The listing builds one solid part. Answer for the finished solid, in the listing's coordinates (mm). A direction names the side the tool comes from. Give positions to 0.01 mm unless a question says otherwise; leave off trailing zeros. Order: outer loops, then holes, each group sorted by start corner. A loop starts at its lowest first (then second) coordinate and runs counter-clockwise, first axis right, second up. Notation, with made-up numbers: (58.25, -19.75) - (112.25, -19.75) arc R25 cw to (112.25, -4.75) - close; hole circle Ø1 at (-14.5, 49.5). An arc over 180 degrees is marked (long way). Write each question's results on one line, items separated by ' | '. Start each with the question number.
1. Determine the mould class of faces 6 (the face through (-69.52, 2.54, 69.82)), 7 (the face through (-67.114, -30, 90)), 8 (the face through (-89, -30, 64.614)) for opening direction Z: released by +Z, released by -Z, zero draft, split by the parting line, or undercut.
2. Which of the six approach directions +Z, -Z, +X, -X, +Y, -Y give full straight-line access (tool end or side, diameter ignored) to faces 1 (the face through (-90, -10, 64.614)), 2 (the face through (-69.36, -9.96, 69.49)), 3 (the face through (-60.858, -18, 91)), 4 (the face through (-46.49, 10.21, 60.63)), 5 (the face through (-64.614, -10, 90))?
3. Section C-C (x = -91) is taken. Give the vertices of the cut face in (y, z).
4. Find the intervals of material crossed by L1, parallel to X at y = -10, z = 94; L2, parallel to Y at x = -71, z = 94; L3, parallel to Z at x = -98, y = -3, in increasing order.
5. Flat-ended cylindrical pins translate along their axes: pin 1 (6 mm diameter, centred on y = 4.5, z = 92, fed in from +X); pin 2 (10 mm diameter, centred on y = 3.5, z = 67.5, fed in from +X); pin 3 (5 mm diameter, centred on y = -10, z = 97.5, fed in from -X); pin 4 (3 mm diameter, centred on x = -89.5, y = -29.5, fed in from -Z). Find the tip coordinate at first contact, or state that the pin passes through.
6. Section D-D (z = 81) is taken. Give the vertices of the cut face in (x, y).
7. Section B-B (z = 96.5) is taken. Give the vertices of the cut face in (x, y), and give its area (3 significant figures).
8. Section A-A (y = -29) is taken. Give the vertices of the cut face in (x, z), and give its area (3 significant figures).
from build123d import *

# Parameters (mm, degrees)
BOSS_EXTRUDE1_DEPTH     = 30
SKETCH2_R               = 2.8
CUT_EXTRUDE1_DEPTH      = 65
CUT_EXTRUDE2_DEPTH      = 65
BOSS_EXTRUDE2_DEPTH     = 40
SKETCH9_W               = 55.910316486
SKETCH9_H               = 20
CUT_EXTRUDE4_DEPTH      = 40
CUT_EXTRUDE5_DEPTH      = 40
CHAMFER1_SIZE           = 5
CUT_EXTRUDE6_DEPTH      = 3
CUT_EXTRUDE6_DEPTH_BACK = 3
CUT_EXTRUDE7_DEPTH      = 3
CUT_EXTRUDE7_DEPTH_BACK = 3
SKETCH14_W              = 8
SKETCH14_H              = 30
BOSS_EXTRUDE3_DEPTH     = 2
CUT_EXTRUDE8_DEPTH      = 22
CHAMFER2_SIZE           = 2


with BuildPart() as part:
    # Sketch1 → Boss-Extrude1 (new body)
    with BuildSketch(Plane(origin=(0, 0, 0), x_dir=(1, 0, 0), z_dir=(0, 1, 0))):
        Polygon((-69, -54.857864376), (-54.857864376, -69), (-39.30151519, -53.443650814), (-33.644660941, -59.100505063), (-49.544155877, -75), (-75, -75), (-75, -49.544155877), (-59.100505063, -33.644660941), (-53.443650814, -39.30151519), align=None)
    extrude(amount=BOSS_EXTRUDE1_DEPTH)

    # Sketch2 → Cut-Extrude1 (cut)
    with BuildSketch(Plane(origin=(12.727922061, 0, 12.727922061), x_dir=(0.707106781, 0, -0.707106781), z_dir=(0.707106781, 0, 0.707106781))):
        with Locations((-70.580735804, 15)):
            Circle(SKETCH2_R)
    extrude(amount=-CUT_EXTRUDE1_DEPTH, mode=Mode.SUBTRACT)

    # Sketch4 → Cut-Extrude2 (cut)
    with BuildSketch(Plane.XZ):
        Polygon((-60.857864376, 75), (-75, 60.857864376), (-82.434342637, 68.292207014), (-68.292207014, 82.434342637), align=None)
    extrude(amount=-CUT_EXTRUDE2_DEPTH, mode=Mode.SUBTRACT)

    # Sketch6 → Boss-Extrude2 (add)
    with BuildSketch(Plane.XZ):
        Polygon((-60.857864376, 75), (-60.857864376, 105.632615689), (-75, 105.632615689), (-75, 75), (-104.149605391, 75), (-104.149605391, 60.857864376), (-75, 60.857864376), (-75, 49.544155877), (-59.100505063, 33.644660941), (-53.443650814, 39.30151519), (-69, 54.857864376), (-54.857864376, 69), (-39.30151519, 53.443650814), (-33.644660941, 59.100505063), (-49.544155877, 75), align=None)
    extrude(amount=BOSS_EXTRUDE2_DEPTH)

    # Sketch9 → Cut-Extrude4 (cut)
    with BuildSketch(Plane(origin=(-61.928932188, 0, 61.928932188), x_dir=(-0.707106781, 0, -0.707106781), z_dir=(0.707106781, 0, -0.707106781))):
        with Locations((0, -30)):
            Rectangle(SKETCH9_W, SKETCH9_H)
    extrude(amount=CUT_EXTRUDE4_DEPTH, mode=Mode.SUBTRACT)

    # Sketch10 → Cut-Extrude5 (cut)
    with BuildSketch(Plane(origin=(12.727922061, 0, 12.727922061), x_dir=(0.707106781, 0, -0.707106781), z_dir=(0.707106781, 0, 0.707106781))):
        Polygon((-87.580735804, -20), (-65.580735804, 0), (-65.580735804, -20), align=None)
    extrude(amount=-CUT_EXTRUDE5_DEPTH, mode=Mode.SUBTRACT)

    # Chamfer1
    chamfer1_edges = [part.edges().sort_by_distance(p)[0] for p in [
        (-67.928932188, 0, 67.928932188),
    ]]
    chamfer(chamfer1_edges, length=CHAMFER1_SIZE)

    # Sketch12 → Cut-Extrude6 (cut, two sides)
    with BuildSketch(Plane(origin=(0, -10, 0), x_dir=(1, 0, 0), z_dir=(0, 1, 0))) as cut_extrude6_sk:
        with BuildLine():
            Line((-75, -67.114451053), (-110.706734673, -67.114451053))
            Line((-110.706734673, -67.114451053), (-110.706734673, -64.614451053))
            Line((-110.706734673, -64.614451053), (-75, -64.614451053))
            ThreePointArc((-75, -64.614451053), (-67.656307913, -67.656307913), (-64.614451053, -75))
            Line((-64.614451053, -75), (-64.614451053, -107.388255064))
            Line((-64.614451053, -107.388255064), (-67.114451053, -107.388255064))
            Line((-67.114451053, -107.388255064), (-67.114451053, -75))
            ThreePointArc((-67.114451053, -75), (-69.424074866, -69.424074866), (-75, -67.114451053))
        make_face()
    extrude(amount=CUT_EXTRUDE6_DEPTH, mode=Mode.SUBTRACT)
    extrude(cut_extrude6_sk.sketch, amount=-CUT_EXTRUDE6_DEPTH_BACK, mode=Mode.SUBTRACT)

    # Sketch13 → Cut-Extrude7 (cut, two sides)
    with BuildSketch(Plane(origin=(0, -30, 0), x_dir=(1, 0, 0), z_dir=(0, 1, 0))) as cut_extrude7_sk:
        with BuildLine():
            Line((-110.706734673, -67.114451053), (-75, -67.114451053))
            ThreePointArc((-75, -67.114451053), (-69.424074866, -69.424074866), (-67.114451053, -75))
            Line((-67.114451053, -75), (-67.114451053, -107.388255064))
            Line((-67.114451053, -107.388255064), (-64.614451053, -107.388255064))
            Line((-64.614451053, -107.388255064), (-64.614451053, -75))
            ThreePointArc((-64.614451053, -75), (-67.656307913, -67.656307913), (-75, -64.614451053))
            Line((-75, -64.614451053), (-110.706734673, -64.614451053))
            Line((-110.706734673, -64.614451053), (-110.706734673, -67.114451053))
        make_face()
    extrude(amount=CUT_EXTRUDE7_DEPTH, mode=Mode.SUBTRACT)
    extrude(cut_extrude7_sk.sketch, amount=-CUT_EXTRUDE7_DEPTH_BACK, mode=Mode.SUBTRACT)

    # Sketch14 → Boss-Extrude3 (add)
    with BuildSketch(Plane(origin=(-46.372583002, 0, 46.372583002), x_dir=(-0.707106781, 0, -0.707106781), z_dir=(0.707106781, 0, -0.707106781))):
        with Locations((-14, 15)):
            Rectangle(SKETCH14_W, SKETCH14_H)
        with Locations((14, 15)):
            Rectangle(SKETCH14_W, SKETCH14_H)
    extrude(amount=BOSS_EXTRUDE3_DEPTH)

    # Sketch15 → Cut-Extrude8 (cut)
    with BuildSketch(Plane(origin=(-20.983069232, 32.641995196, 20.983069232), x_dir=(0.879633819, 0.400113768, 0.257202871), z_dir=(0.475651494, -0.739940073, -0.475651494))):
        Polygon((-16.653515894, 59.58496844), (-53.507538304, 34.603245183), (-43.108288721, 19.261862476), (-6.254266311, 44.243585732), align=None)
    extrude(amount=CUT_EXTRUDE8_DEPTH, mode=Mode.SUBTRACT)

    # Chamfer2
    chamfer2_edges = [part.edges().sort_by_distance(p)[0] for p in [
        (-60.857864376, -17.5, 75),
        (-75, -17.5, 60.857864376),
    ]]
    chamfer(chamfer2_edges, length=CHAMFER2_SIZE)


solid = part.part
Reported:
1) face 6: released by +Z | face 7: zero draft | face 8: undercut
2) face 1: -X | face 2: none | face 3: +Z, +X, +Y, -Y | face 4: +Y, -Y | face 5: +Z
3) outline: (-40, 60.86) - (0, 60.86) - (0, 75) - (-40, 75) - close; hole (-33, 64.61) - (-27, 64.61) - (-27, 67.11) - (-33, 67.11) - close; hole (-13, 64.61) - (-7, 64.61) - (-7, 67.11) - (-13, 67.11) - close
4) L1: -75 to -67.11, -64.61 to -60.86 | L2: -40 to 0 | L3: 60.86 to 75
5) pin 1: through | pin 2: x = -37.04 | pin 3: x = -75 | pin 4: z = 60.86
6) outline: (-75, -40) - (-60.86, -40) - (-60.86, 0.76) - (-61.93, 0) - (-75, 0) - close; hole (-67.11, -33) - (-64.61, -33) - (-64.61, -27) - (-67.11, -27) - close; hole (-67.11, -13) - (-64.61, -13) - (-64.61, -7) - (-67.11, -7) - close
7) outline: (-75, -40) - (-60.86, -40) - (-60.86, 0) - (-75, 0) - close; hole (-67.11, -33) - (-64.61, -33) - (-64.61, -27) - (-67.11, -27) - close; hole (-67.11, -13) - (-64.61, -13) - (-64.61, -7) - (-67.11, -7) - close | area: 536 mm²
8) outline: (-104.15, 60.86) - (-77, 60.86) - (-75, 58.86) - (-75, 49.54) - (-74.66, 49.2) - (-49.2, 74.66) - (-49.54, 75) - (-58.86, 75) - (-60.86, 77) - (-60.86, 105.63) - (-64.61, 105.63) - (-64.61, 75) arc R10.39 cw to (-75, 64.61) - (-104.15, 64.61) - close; (-104.15, 67.11) - (-75, 67.11) arc R7.89 ccw to (-67.11, 75) - (-67.11, 105.63) - (-75, 105.63) - (-75, 75) - (-104.15, 75) - close | area: 1,010 mm²
